Here's the drawing with two shaded views (mm, measured from the low corner). I have some questions. Give positions to 0.01 mm unless a question says otherwise; leave off trailing zeros. Write each loop counter-clockwise with the first axis right and the second up, starting at its lowest first coordinate (ties: lowest second). Pieces come first, ordered by that corner, then holes.
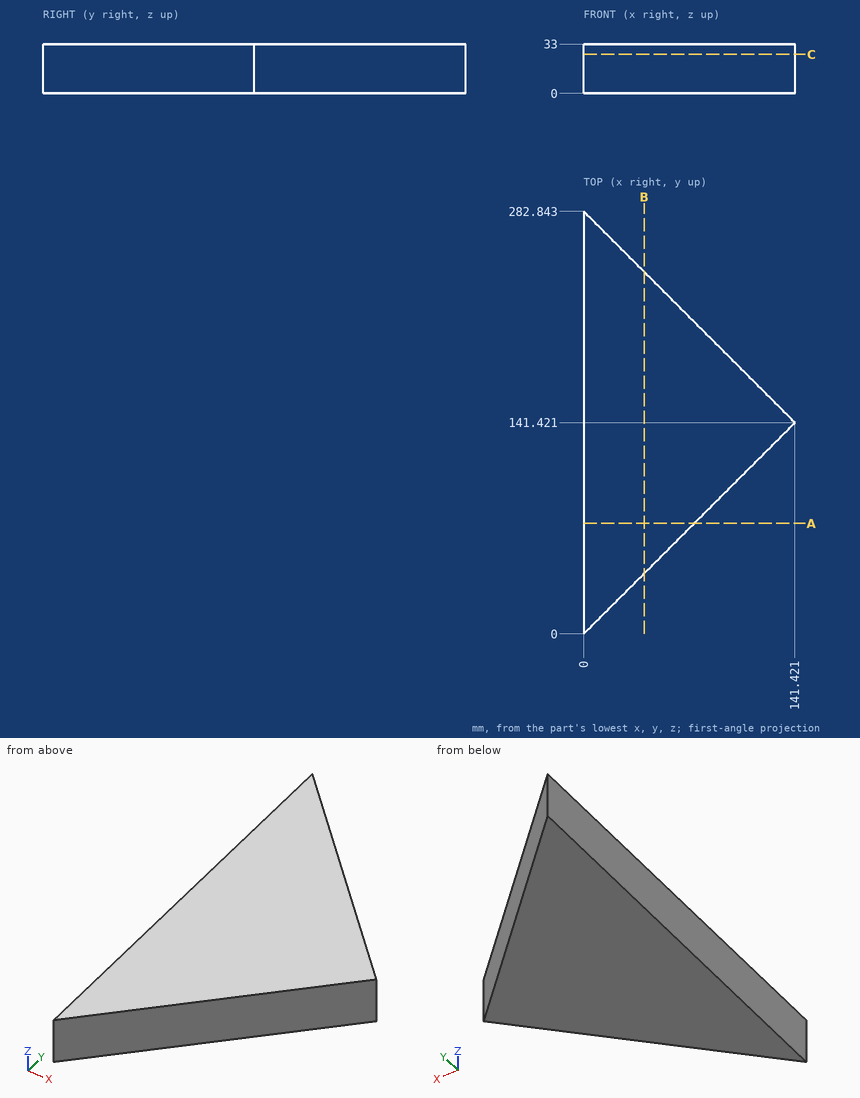
(1) Will these pins go through, and if not, where does the flat tip stop? P1, Ø6, axis at x = 89.5, z = 11.5, coming from the +Y side; P2, Ø1.5, axis at x = 112, z = 22, coming from the +Y side; P3, Ø2, axis at y = 82, z = 20.5, coming from the +X side.
Returned:
P1: stops at y = 196.34
P2: stops at y = 171.59
P3: stops at x = 83
(2) Imagine slicing it at B-B, the plane x = 40.5. Write out the boundary of the cut face in (y, z).
Returned:
outline: (40.5, 0) - (242.34, 0) - (242.34, 33) - (40.5, 33) - close
(3) If I drill on L1, parallel to Y at x = 59, z = 18.5; L2, parallel to Y at x = 41.5, z = 14; L3, parallel to X at y = 189.5, z = 28, over which ranges is the centre line in solid material (lowest first)?
Returned:
L1: y = 59 to 223.84
L2: y = 41.5 to 241.34
L3: x = 0 to 93.34
(4) Imagine slicing it at C-C, the plane z = 26. Write out the boundary of the cut face in (x, y), plus the area to 3 significant figures.
Returned:
outline: (0, 0) - (141.42, 141.42) - (0, 282.84) - close
area: 20,000 mm2
(5) Imagine slicing it at A-A, the plane y = 74. Write out the boundary of the cut face in (x, z), plus the area to 3 significant figures.
Returned:
outline: (0, 0) - (74, 0) - (74, 33) - (0, 33) - close
area: 2,440 mm2
